Read the model definition and answer for the solid it produces. Units are mm, in the model's axes. A direction names the side the tool comes from. Give positions to 0.01 mm unless a question says otherwise; leave off trailing zeros. Write each loop counter-clockwise with the first axis right and the second up, starting at its lowest first coordinate (ties: lowest second). Pieces come first, ordered by that corner, then holes. Notation, with made-up numbers: (2, -26) -> (12, -26) arc R32 ccw to (12, 8) -> close; hole circle Ø8 at (26, -8.75). An arc over 180 degrees is marked (long way). Put each result on its own line as item: value. Start each with the question number.
from build123d import *

# Parameters (mm, degrees)
F1_DEPTH = 32
F2_R     = 6
F3_DEPTH = 25
F6_DEPTH = 1000


with BuildPart() as f1:
    # F0 (on Front) → F1 (new body, symmetric)
    with BuildSketch(Plane.XZ):
        Polygon((-58.409637, 26), (-58.409637, 0), (-40.409637, 0), (-40.409637, 12), (37.590363, 12), (37.590363, 0), (55.590363, 0), (55.590363, 26), align=None)
    extrude(amount=F1_DEPTH, both=True)

    # F2 (on face) → F3 (cut)
    with BuildSketch(Plane.XY.offset(26)):
        with Locations((-34.409637, 0)):
            Circle(F2_R)
    extrude(amount=-F3_DEPTH, mode=Mode.SUBTRACT)

    # F5 (on face) → F6 (cut)
    with BuildSketch(Plane.YZ.offset(55.590363)):
        Polygon((-14, 0), (0, 0), (14, 0), (20, 12), (0, 12), (-20, 12), align=None)
    extrude(amount=-F6_DEPTH, mode=Mode.SUBTRACT)


solid = f1.part
1) A cutting plane is placed at C-C on y = 16. Give the vertices of the cut face in (x, z), and give its area (3 significant figures).
2) A cutting plane is placed at D-D on x = -32.5. Give the vertices of the cut face in (y, z).
3) For a pull along Z with two mould halves and no side action, classify faces 4 (the face through (-50, -23, 0)), 5 (the face through (-1, 0, 26)), 6 (the face through (-49, 17, 6)), 7 (the face through (-58.41, 0, 16)) as pulls with the +Z half, pulls with the -Z half, needs draft (parallel to the pull), parting line crosses it, or undercut.
4) A cutting plane is placed at A-A on y = 0. Give the vertices of the cut face in (x, z), and give its area (3 significant figures).
5) For faces 1 (the face through (-50, 23, 0)), 2 (the face through (47, 17, 6)), 3 (the face through (-40.41, 25, 6)), determine the directions among +Z, -Z, +X, -X, +Y, -Y from which every point of the face is accessible in a straight line to the end or side of a thin tool.
6) This flat-tipped pin is pushed along its axis until it touches: pin 1 Ø1 at (x, y) = (-25, -12.5) entering from -Z. Where does it stop, or does it pass through?
7) A cutting plane is placed at B-B on z = 7.5. Give the vertices of the cut face in (x, y), and give its area (3 significant figures).
8) Straight lines are drawn through the part: line 1 (Z direction, x = -3.5, y = 0); line 2 (Y direction, x = -52.5, z = 5.5); line 3 (Y direction, x = 51, z = 10.5). For each, find the intervals that lie inside material, in ascending order. Write a range as [from, to].
Results found:
1. outline: (-58.41, 0) -> (-40.41, 0) -> (-40.41, 4) -> (-58.41, 4) -> close; (-58.41, 12) -> (55.59, 12) -> (55.59, 26) -> (-58.41, 26) -> close; (37.59, 0) -> (55.59, 0) -> (55.59, 4) -> (37.59, 4) -> close
1. area: 1,740 mm²
2. outline: (-32, 12) -> (-5.69, 12) -> (-5.69, 26) -> (-32, 26) -> close; (5.69, 12) -> (32, 12) -> (32, 26) -> (5.69, 26) -> close
3. face 4: pulls with the -Z half
3. face 5: pulls with the +Z half
3. face 6: undercut
3. face 7: needs draft
4. outline: (-58.41, 12) -> (-40.41, 12) -> (-40.41, 26) -> (-58.41, 26) -> close; (-28.41, 12) -> (55.59, 12) -> (55.59, 26) -> (-28.41, 26) -> close
4. area: 1,430 mm²
5. face 1: -Z, +X, -X, +Y, -Y
5. face 2: +X, -X
5. face 3: -Z, +Y, -Y
6. pin 1: stops at z = 12
7. outline: (-58.41, -32) -> (-40.41, -32) -> (-40.41, -17.75) -> (-58.41, -17.75) -> close; (-58.41, 17.75) -> (-40.41, 17.75) -> (-40.41, 32) -> (-58.41, 32) -> close; (37.59, -32) -> (55.59, -32) -> (55.59, -17.75) -> (37.59, -17.75) -> close; (37.59, 17.75) -> (55.59, 17.75) -> (55.59, 32) -> (37.59, 32) -> close
7. area: 1,030 mm²
8. line 1: z = [12, 26]
8. line 2: y = [-32, -16.75], [16.75, 32]
8. line 3: y = [-32, -19.25], [19.25, 32]
